Geometry: final body of the model. Coordinates: model frame, mm. Face numbers are marked on the shaded views. A direction names the side the tool comes from. Give positions to 0.01 mm unless a question says otherwise; leave off trailing zeros. Order: outer loops, then holes, each group sorted by start corner. A loop starts at its lowest first (then second) coordinate and runs counter-clockwise, first axis right, second up. Notation, with made-up numbers: (11.25, -36.5) - (23.25, -36.5) arc R13 ccw to (23.25, -12.5) - close; hole circle Ø3 at (38, 2). An arc over 180 degrees is marked (long way). Put each result on its own line as item: value. Start each with the question number.
1. Mould query, pull axis X, two halves, no side actions, for the marked faces 5, 6, 7 and 8. Classes: pulls with the +X half, pulls with the -X half, needs draft (parallel to the pull), parting line crosses it, or undercut.
2. Section D-D on z = 25.5. Return the cut outline in (x, y), plus the area to 3 significant figures.
3. Section C-C on y = -2. Return the cut outline in (x, z), plus the area to 3 significant figures.
4. First-contact query: P1, Ø12, axis at x = 5, y = -17, coming from the -Z side; P2, Ø1, axis at x = -21.5, z = 19.5, coming from the +Y side; P3, Ø10, axis at x = -18.5, z = 25.5, coming from the -Y side; P4, Ø5.5, axis at x = -28, z = 32, coming from the -Y side. Flat tips, straight axial feed; report the tip coordinate or a pass-through.
5. Section B-B on y = 87.25. Return the cut outline in (x, z).
6. Ray query, line 1 along Z through (x, y) = (9.5, 52.5); line 2 along X through (y, z) = (-15.5, 12); line 3 along Y through (x, z) = (-21.5, 31). Return the intervals inside material, ascending. Write a range as from..to.
7. Set-up query: the marked faces 1, 2, 3 and 4. Return all of +Z, -Z, +X, -X, +Y, -Y with unobstructed straight access to the full face (end or side cutting, diameter ignored); none if empty.
8. Section A-A on x = -6. Return the cut outline in (y, z), plus the area to 3 significant figures.
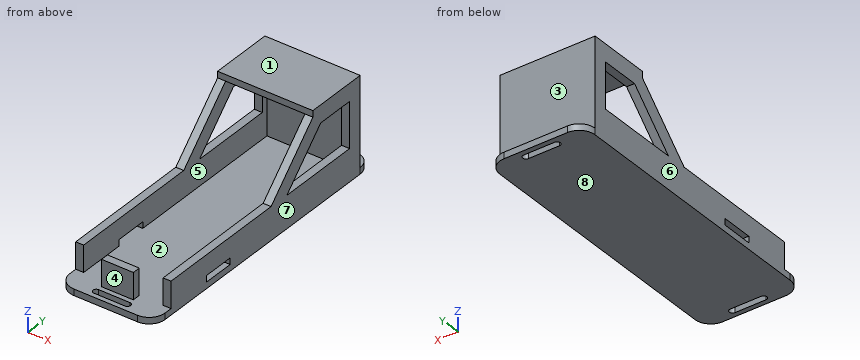
from build123d import *

# Parameters (mm, degrees)
SALIENTE_EXTRUIR2_DEPTH    = 4
SALIENTE_EXTRUIR3_DEPTH    = 52
CROQUIS3_W                 = 60
CROQUIS3_H                 = 4
SALIENTE_EXTRUIR4_DEPTH    = 40
CORTAR_EXTRUIR1_DEPTH      = 87
CORTAR_EXTRUIR2_DEPTH      = 87
CORTAR_EXTRUIR2_DEPTH_BACK = 87
CROQUIS6_W                 = 4
CROQUIS6_H                 = 20
CORTAR_EXTRUIR3_DEPTH      = 87
CORTAR_EXTRUIR4_DEPTH      = 87


with BuildPart() as part:
    # Croquis1 → Saliente-Extruir2 (new body)
    with BuildSketch(Plane.XY):
        with BuildLine():
            ThreePointArc((-30, 82.5), (-27.071067812, 89.571067812), (-20, 92.5))
            Line((-20, 92.5), (20, 92.5))
            ThreePointArc((20, 92.5), (27.071067812, 89.571067812), (30, 82.5))
            Line((30, 82.5), (-30, 82.5))
        make_face()
        Polygon((25, 77.5), (25, -77.5), (30, -77.5), (30, 82.5), (-30, 82.5), (-30, -77.5), (-25, -77.5), (-25, 77.5), align=None)
        Polygon((-10, -77.5), (0, -77.5), (10, -77.5), (25, -77.5), (25, 77.5), (-25, 77.5), (-25, -77.5), align=None)
        with BuildLine():
            Line((25, -77.5), (10, -77.5))
            Line((10, -77.5), (10, -82.5))
            Line((10, -82.5), (-10, -82.5))
            Line((-10, -82.5), (-10, -77.5))
            Line((-10, -77.5), (-25, -77.5))
            Line((-25, -77.5), (-30, -77.5))
            Line((-30, -77.5), (-30, -82.5))
            ThreePointArc((-30, -82.5), (-27.071067812, -89.571067812), (-20, -92.5))
            Line((-20, -92.5), (20, -92.5))
            ThreePointArc((20, -92.5), (27.071067812, -89.571067812), (30, -82.5))
            Line((30, -82.5), (30, -77.5))
            Line((30, -77.5), (25, -77.5))
        make_face()
        Polygon((10, -77.5), (0, -77.5), (-10, -77.5), (-10, -82.5), (10, -82.5), align=None)
    extrude(amount=SALIENTE_EXTRUIR2_DEPTH)

    # Croquis2 → Saliente-Extruir3 (add)
    with BuildSketch(Plane.XY.offset(4)):
        Polygon((10, -77.5), (0, -77.5), (-10, -77.5), (-10, -82.5), (10, -82.5), align=None)
        Polygon((25, 77.5), (25, -77.5), (30, -77.5), (30, 82.5), (-30, 82.5), (-30, -77.5), (-25, -77.5), (-25, 77.5), align=None)
    extrude(amount=SALIENTE_EXTRUIR3_DEPTH)

    # Croquis3 → Saliente-Extruir4 (add)
    with BuildSketch(Plane(origin=(0, 82.5, 0), x_dir=(1, 0, 0), z_dir=(0, 1, 0))):
        with Locations((0, -58)):
            Rectangle(CROQUIS3_W, CROQUIS3_H)
    extrude(amount=-SALIENTE_EXTRUIR4_DEPTH)

    # Croquis4 → Cortar-Extruir1 (cut)
    with BuildSketch(Plane.ZY.offset(30)):
        Polygon((56, 42.5), (20.644660941, 7.144660941), (20.644660941, -100.088523904), (56, -100.088523904), align=None)
    extrude(amount=-CORTAR_EXTRUIR1_DEPTH, mode=Mode.SUBTRACT)

    # Croquis6 → Cortar-Extruir2 (cut, two sides: drawn at the far end of the back side and taken through both)
    with BuildSketch(Plane.ZY.offset(-25).offset(-CORTAR_EXTRUIR2_DEPTH_BACK)):
        with Locations((6, -37.5)):
            Rectangle(CROQUIS6_W, CROQUIS6_H)
    extrude(amount=CORTAR_EXTRUIR2_DEPTH + CORTAR_EXTRUIR2_DEPTH_BACK, mode=Mode.SUBTRACT)

    # Croquis7 → Cortar-Extruir3 (cut)
    with BuildSketch(Plane.ZY.offset(30)):
        Polygon((20.325435978, 20.468039644), (20.325435978, 73.545906874), (48.990760507, 73.545906874), (48.990760507, 49.133364172), align=None)
    extrude(amount=-CORTAR_EXTRUIR3_DEPTH, mode=Mode.SUBTRACT)

    # Croquis8 → Cortar-Extruir4 (cut)
    with BuildSketch(Plane.XY.offset(4)):
        with BuildLine():
            Line((-9.602247867, -85.5), (10, -85.5))
            ThreePointArc((10, -85.5), (12, -87.5), (10, -89.5))
            Line((10, -89.5), (-9.602247867, -89.5))
            ThreePointArc((-9.602247867, -89.5), (-11.602247867, -87.5), (-9.602247867, -85.5))
        make_face()
        with BuildLine():
            Line((10, 85.25), (-9.602247867, 85.25))
            ThreePointArc((-9.602247867, 85.25), (-11.602247867, 87.25), (-9.602247867, 89.25))
            Line((-9.602247867, 89.25), (10, 89.25))
            ThreePointArc((10, 89.25), (12, 87.25), (10, 85.25))
        make_face()
    extrude(amount=-CORTAR_EXTRUIR4_DEPTH, mode=Mode.SUBTRACT)


solid = part.part
Resolved:
1. face 5: undercut
1. face 6: pulls with the -X half
1. face 7: pulls with the +X half
1. face 8: needs draft
2. outline: (-30, 12) - (-25, 12) - (-25, 25.64) - (-30, 25.64) - close; (-30, 73.55) - (-25, 73.55) - (-25, 77.5) - (25, 77.5) - (25, 73.55) - (30, 73.55) - (30, 82.5) - (-30, 82.5) - close; (25, 12) - (30, 12) - (30, 25.64) - (25, 25.64) - close
2. area: 476 mm^2
3. outline: (-30, 0) - (30, 0) - (30, 20.64) - (25, 20.64) - (25, 4) - (-25, 4) - (-25, 20.64) - (-30, 20.64) - close
3. area: 406 mm^2
4. P1: z = 0
4. P2: y = 82.5
4. P3: y = 77.5
4. P4: y = 15.75
5. outline: (-28.8, 0) - (-11.6, 0) - (-11.6, 4) - (-28.8, 4) - close; (12, 0) - (28.8, 0) - (28.8, 4) - (12, 4) - close
6. line 1: 0..4, 56..60
6. line 2: -30..-25, 25..30
6. line 3: 77.5..82.5
7. face 1: +Z, +X, -X, +Y, -Y
7. face 2: none
7. face 3: +Z, +X, -X, +Y
7. face 4: +Z, +X, -X, -Y
8. outline: (-92.5, 0) - (-89.5, 0) - (-89.5, 4) - (-92.5, 4) - close; (-85.5, 0) - (85.25, 0) - (85.25, 4) - (82.5, 4) - (82.5, 60) - (42.5, 60) - (42.5, 56) - (77.5, 56) - (77.5, 4) - (-77.5, 4) - (-77.5, 20.64) - (-82.5, 20.64) - (-82.5, 4) - (-85.5, 4) - close; (89.25, 0) - (92.5, 0) - (92.5, 4) - (89.25, 4) - close
8. area: 1,210 mm^2
